Autodesk Inventor part; units mm, degrees
ref_plane "YZ Plane" through (0, 0, 0) normal (1, 0, 0) x (0, 1, 0)
ref_plane "XZ Plane" through (0, 0, 0) normal (0, 1, 0) x (-1, 0, 0)
ref_plane "XY Plane" through (0, 0, 0) normal (0, 0, 1) x (1, 0, 0)
sketch "Sketch1" plane through (0, 0, 0) normal (0, 0, 1) x (1, 0, 0)
  line L0 (0, 0) -> (16, 0)
  line L1 (16, 0) -> (16, 10)
  line L2 (16, 10) -> (0, 10)
  line L3 (0, 10) -> (0, 0)
  dimension "d0" = 16
  dimension "d1" = 10
extrude "Extrusion1" add sketch "Sketch1" along normal blind 2
sketch "Sketch2" plane through (0, 0, 2) normal (0, 0, 1) x (1, 0, 0)
  line L0 (0, 0) -> (0, 10)
  line L1 (16, 0) -> (0, 0)
  line L2 (16, 10) -> (16, 0)
  line L3 (0, 10) -> (16, 10)
  line L4 (1.1176, 8.8824) -> (1.1176, 1.1176)
  line L5 (1.1176, 1.1176) -> (14.8824, 1.1176)
  line L6 (14.8824, 1.1176) -> (14.8824, 8.8824)
  line L7 (14.8824, 8.8824) -> (1.1176, 8.8824)
  dimension "d4" = 1.1176
extrude "Extrusion2" cut sketch "Sketch2" against normal blind 1
sketch "Sketch3" plane through (0, 10, 0) normal (0, 1, 0) x (1, 0, 0)
  line L0 (0, -1) -> (16, -1)
  line L1 (16, 0) -> (0, 0)
  line L2 (0, 0) -> (0, -1)
  line L3 (6, 0) -> (10, 0)
  line L4 (10, 0) -> (10, -1)
  line L5 (10, -1) -> (6, -1)
  line L6 (6, -1) -> (6, 0)
  dimension "d7" = 4
  dimension "d8" = 6
extrude "Extrusion3" add sketch "Sketch3" along normal blind 4 contours L6 L1 L4 L0
sketch "Sketch4" plane through (0, 0, 1) normal (0, 0, 1) x (1, 0, 0)
  point P0 (8, 12)
hole "Hole1" at (8, 12, 1) direction (0, 0, -1) diameter 1.905 end through all
fillet "Fillet1" radius 0.5 12 edges at (1.1176, 1.1176, 1.5) (0, 0, 0.5) (1.1176, 8.8824, 1.5) (0, 10, 0.5) (14.8824, 1.1176, 1.5) (16, 0, 0.5) (14.8824, 8.8824, 1.5) (16, 10, 0.5) (10, 10, 0.5) (6, 10, 0.5) (6, 14, 0.5) (10, 14, 0.5)
properties part number "lid"
Could you check a few things on this model? Use its own coordinates, in mm. A direction names the side the tool comes from. Give positions to 0.01 mm unless a question says otherwise; leave off trailing zeros. Order: outer loops, then holes, each group sorted by start corner. A loop starts at its lowest first (then second) coordinate and runs counter-clockwise, first axis right, second up.
Q1. For faces 1 (the flat face through (7.9, 1.118, 1.5)), 2 (the flat face through (14.882, 5, 1.5)), 3 (the flat face through (8.1, 8.882, 1.5)), 4 (the flat face through (13, 10, 0.5)), which set-ups out of +Z, -Z, +X, -X, +Y, -Y let a thin tool reach every point of the face, with its end or its side?
Q2. Suppose I cut it at B-B, the plane x = 8. Write out the boundary of the cut face in (y, z), and give its area (3 significant figures).
Q3. We'd pull the mould along X, two halves only. Please class faces 5 (the cylindrical face through (8.36, 11.12, 0.49)), 6 (the flat face through (3, 10, 0.5)), 7 (the flat face through (16, 4.9, 0.5)), 8 (the flat face through (1.118, 5, 1.5)): +X half, -X half, draft (parallel to the pull), parting line (faces both ways), or undercut.
Q4. I'm going to push flat-ended pins straight in: P1, Ø1.1, axis at y = 12, z = 0.5, coming from the +X side; P2, Ø0.8, axis at x = 2, z = 0.5, coming from the +Y side; P3, Ø1.5, axis at x = 8, y = 12, coming from the -Z side; P4, Ø0.5, axis at x = 8.5, z = 1.5, coming from the -Y side. Where does each tip first touch, or does it pass through?
Q5. Suppose I cut it at C-C, the plane y = 12. Write out the boundary of the cut face in (x, z).
Q6. If I drill on line 1 along X through (y, z) = (12, 0.7); line 2 along Y through (x, z) = (8, 0.7); line 3 along Z through (x, y) = (7.5, 10), over which ranges is the centre line in solid material (lowest first)?
Q7. Suppose I cut it at A-A, the plane z = 0.65. Write out the boundary of the cut face in (x, y) (1 decimal), and give its area (3 significant figures).
Q8. Suppose I cut it at D-D, the plane z = 1.65. Write out the boundary of the cut face in (x, y), and give its area (3 significant figures).
Solution:
1. face 1: +Z, +X, -X, -Y
1. face 2: +Z, +X, +Y, -Y
1. face 3: +Z, +X, -X, +Y
1. face 4: +Z, -Z, +X, +Y
2. outline: (0, 0) - (11.05, 0) - (11.05, 1) - (8.88, 1) - (8.88, 2) - (1.12, 2) - (1.12, 1) - (0, 1) - close; (12.95, 0) - (14, 0) - (14, 1) - (12.95, 1) - close
2. area: 19.9 mm2
3. face 5: undercut
3. face 6: draft
3. face 7: +X half
3. face 8: -X half
4. P1: stops at x = 10
4. P2: stops at y = 10
4. P3: passes through
4. P4: stops at y = 1.12
5. outline: (6, 0) - (7.05, 0) - (7.05, 1) - (6, 1) - close; (8.95, 0) - (10, 0) - (10, 1) - (8.95, 1) - close
6. line 1: x = 6 to 7.05, 8.95 to 10
6. line 2: y = 0 to 11.05, 12.95 to 14
6. line 3: z = 0 to 1
7. outline: (0, 0.5) arc R0.5 ccw to (0.5, 0) - (15.5, 0) arc R0.5 ccw to (16, 0.5) - (16, 9.5) arc R0.5 ccw to (15.5, 10) - (10.5, 10) arc R0.5 cw to (10, 10.5) - (10, 13.5) arc R0.5 ccw to (9.5, 14) - (6.5, 14) arc R0.5 ccw to (6, 13.5) - (6, 10.5) arc R0.5 cw to (5.5, 10) - (0.5, 10) arc R0.5 ccw to (0, 9.5) - close; hole circle Ø1.9 at (8, 12)
7. area: 173 mm2
8. outline: (1.12, 1.62) arc R0.5 ccw to (1.62, 1.12) - (14.38, 1.12) arc R0.5 ccw to (14.88, 1.62) - (14.88, 8.38) arc R0.5 ccw to (14.38, 8.88) - (1.62, 8.88) arc R0.5 ccw to (1.12, 8.38) - close
8. area: 107 mm2
